For this review, use the dimensioned drawing (mm, ordinates from the lowest corner) and the shaded views. A direction names the side the tool comes from. Give positions to 0.01 mm unless a question says otherwise; leave off trailing zeros. Loops run counter-clockwise (first coordinate to the right, second up) from the corner with the lowest first, then second, coordinate; pieces in that order, holes last. Notation, with made-up numbers: (31, 68) - (57, 68) arc R27 cw to (57, 99) - close; hole circle Ø8 at (-3.75, 7). An arc over 180 degrees is marked (long way). Put each result on its own line as item: value.
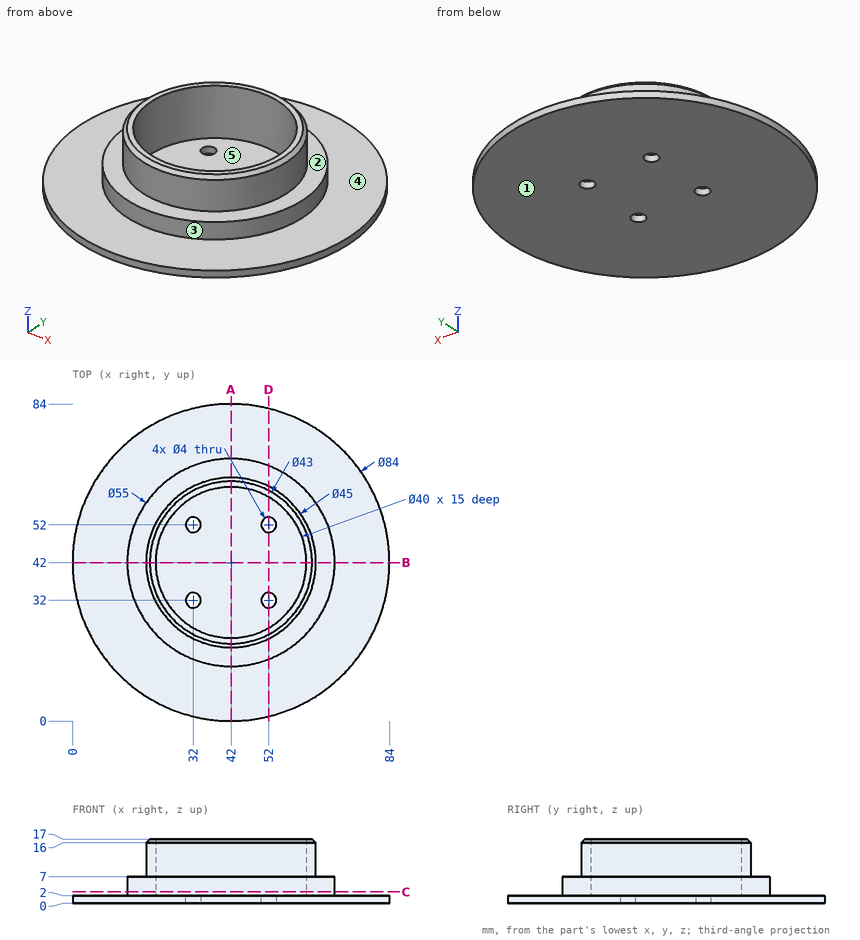
1) Draft analysis for pull direction Y (two halves, no side actions). For the marked faces 3, 4 and 5, state which applies: pulls with the +Y half, pulls with the -Y half, needs draft (parallel to the pull), parting line crosses it, or undercut.
Geometry check:
face 3: parting line crosses it
face 4: needs draft
face 5: undercut
2) For the marked faces 1 and 2, list the 3-axis set-ups (+Z, -Z, +X, -X, +Y, -Y) from which the entire face can be reached by the end or side of a thin tool; tool diameter is ignored.
Geometry check:
face 1: -Z, +X, -X, +Y, -Y
face 2: +Z
3) Take a section at A-A on x = 42. State the section outline as (y, z) points, and give its area (3 significant figures).
Geometry check:
outline: (0, 0) - (84, 0) - (84, 2) - (69.5, 2) - (69.5, 7) - (64.5, 7) - (64.5, 16) - (63.5, 17) - (62, 17) - (62, 2) - (22, 2) - (22, 17) - (20.5, 17) - (19.5, 16) - (19.5, 7) - (14.5, 7) - (14.5, 2) - (0, 2) - close
area: 292 mm²
4) Insertion check: pin 1 Ø2.5 at (x, y) = (52, 52) entering from +Z; pin 2 Ø5 at (x, y) = (32, 32) entering from -Z; pin 3 Ø4 at (y, z) = (48.5, 7.5) entering from -X; pin 4 Ø1.5 at (y, z) = (29.5, 9.5) entering from -X. Each pin has a flat end and moves straight along its axis. Give the tip position at first contact, or say it passes through.
Geometry check:
pin 1: passes through
pin 2: stops at z = 0
pin 3: stops at x = 14.88
pin 4: stops at x = 22.81
5) Take a section at D-D on x = 52. State how many separate pieces and enclosed holes the cut face has, and give its area (3 significant figures).
Geometry check:
separate pieces: 3
enclosed holes: 0
area: 286 mm²
6) Take a section at C-C on z = 3. State the section outline as (x, y) points.
Geometry check:
outline: circle Ø55 at (42, 42); hole circle Ø40 at (42, 42)
7) Wall thickness on line 1 (Y direction, x = 52, z = 0.95); line 2 (Z direction, x = 23, y = 10); line 3 (X direction, y = 48, z = 10): over which ranges is each line inside the solid? List them lowest first.
Geometry check:
line 1: y = 1.21 to 30, 34 to 50, 54 to 82.79
line 2: z = 0 to 2
line 3: x = 20.31 to 22.92, 61.08 to 63.69
